Could you check a few things on this model? Use its own coordinates, in mm. Face numbers are marked on the shaded views. Give positions to 0.01 mm unless a question says otherwise; leave off trailing zeros. Order: outer loops, then holes, each group sorted by start corner. A loop starts at its lowest first (then second) coordinate and runs counter-clockwise, first axis right, second up. Notation, with made-up numbers: (-18, 48.25) - (18, 48.25) arc R33 cw to (18, 82.25) - close; hole circle Ø1 at (-6.5, 28). An arc over 180 degrees is marked (long way). Put each result on its own line as item: value.
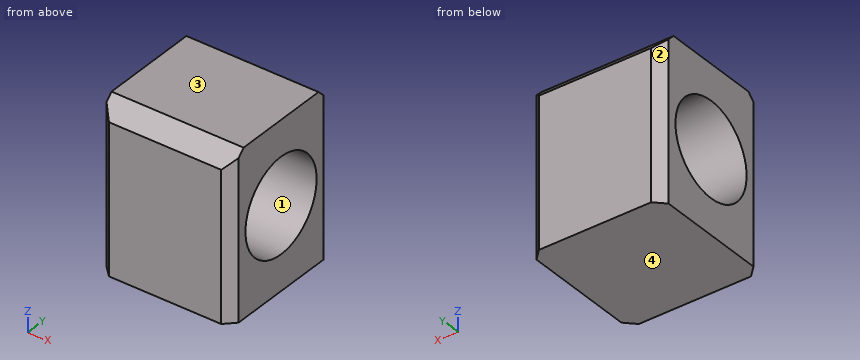
Autodesk Inventor part; units mm, degrees
ref_plane "YZ Plane" through (0, 0, 0) normal (1, 0, 0) x (0, 1, 0)
ref_plane "XZ Plane" through (0, 0, 0) normal (0, 1, 0) x (-1, 0, 0)
ref_plane "XY Plane" through (0, 0, 0) normal (0, 0, 1) x (1, 0, 0)
sketch "Sketch1" plane through (0, 0, 0) normal (0, 0, 1) x (1, 0, 0)
  line L0 (40, 40) -> (40, -40)
  line L1 (40, -40) -> (-40, -40)
  line L2 (-40, -40) -> (-40, 40)
  line L3 (-40, 40) -> (40, 40)
  point P0 (0, 0)
  point P1 (0, 0)
  dimension "d0" = 80
extrude "Extrusion1" add sketch "Sketch1" along normal blind 100
sketch "Sketch2" plane through (-40, -40, 0) normal (-1, 0, 0) x (0, 0, 1)
  line L0 (100, 0) -> (100, 80)
  line L1 (0, 80) -> (100, 80)
  point P0 (50, 40)
  dimension "d3" = 50
  dimension "d4" = 40
hole "Hole1" at (-40, 0, 50) direction (1, 0, 0) diameter 57 end through all
chamfer "Chamfer2" distance 10 angle 45 2 edges at (0, -40, 100) (0, 40, 100)
chamfer "Chamfer1" distance 6 angle 45 4 edges at (-40, 40, 45) (40, 40, 45) (-40, -40, 45) (40, -40, 45)
properties part number "3136 1094 56" material "Steel, Mild"
1) If I drill on line 1 (Z direction, x = -2, y = 0); line 2 (Y direction, x = 2.5, z = 50); line 3 (Z direction, x = 10.5, y = 20.5), over which ranges is the centre line in solid material (lowest first)? Write a range as [from, to].
Filled in:
line 1: z = [0, 21.5], [78.5, 100]
line 2: y = [-40, -28.5], [28.5, 40]
line 3: z = [0, 30.2], [69.8, 100]
2) Suppose I cut it at A-A, the plane z = 50. List the corners of the cut face in (x, y) for me, and give its area (3 significant figures).
Filled in:
outline: (-40, -34) - (-34, -40) - (34, -40) - (40, -34) - (40, -28.5) - (-40, -28.5) - close; (-40, 28.5) - (40, 28.5) - (40, 34) - (34, 40) - (-34, 40) - (-40, 34) - close
area: 1,770 mm^2
3) Suppose I cut it at B-B, the plane y = 0. List the corners of the cut face in (x, z) for me.
Filled in:
outline: (-40, 0) - (40, 0) - (40, 21.5) - (-40, 21.5) - close; (-40, 78.5) - (40, 78.5) - (40, 100) - (-40, 100) - close
4) Suppose I cut it at D-D, the plane y = -24. List the corners of the cut face in (x, z) for me, and give its area (3 significant figures).
Filled in:
outline: (-40, 0) - (40, 0) - (40, 34.63) - (-40, 34.63) - close; (-40, 65.37) - (40, 65.37) - (40, 100) - (-40, 100) - close
area: 5,540 mm^2
5) We'd pull the mould along Z, two halves only. Please class the marked faces 1, 2, 3 and 4: pulls with the +Z half, pulls with the -Z half, needs draft (parallel to the pull), parting line crosses it, or undercut.
Filled in:
face 1: undercut
face 2: needs draft
face 3: pulls with the +Z half
face 4: pulls with the -Z half
6) Suppose I cut it at C-C, the plane x = 8. List the corners of the cut face in (y, z) for me, and give its area (3 significant figures).
Filled in:
outline: (-40, 0) - (40, 0) - (40, 90) - (30, 100) - (-30, 100) - (-40, 90) - close; hole circle Ø57 at (0, 50)
area: 5,350 mm^2
7) I'm going to push a flat-ended pin straight in: pin 1 (1 mm diameter, centred on x = 22.5, y = -24, fed in from -Z). Where does the tip first touch, or does it pass through?
Filled in:
pin 1: stops at z = 0
